```python
from build123d import *

# Parameters (mm, degrees)
SKETCH1_W           = 50
SKETCH1_H           = 50
BOSS_EXTRUDE1_DEPTH = 50
SKETCH2_R           = 20
CUT_EXTRUDE1_DEPTH  = 5
SKETCH3_R           = 20
CUT_EXTRUDE5_DEPTH  = 2
FILLET10_R          = 30
FILLET11_R          = 10
FILLET12_R          = 10
FILLET15_R          = 5
FILLET16_R          = 5


with BuildPart() as part:
    # Sketch1 → Boss-Extrude1 (new body)
    with BuildSketch(Plane(origin=(0, 0, 0), x_dir=(1, 0, 0), z_dir=(0, 1, 0))):
        Rectangle(SKETCH1_W, SKETCH1_H)
    extrude(amount=BOSS_EXTRUDE1_DEPTH)

    # Sketch2 → Cut-Extrude1 (cut)
    with BuildSketch(Plane(origin=(0, 0, -25), x_dir=(-1, 0, 0), z_dir=(0, 0, -1))):
        with Locations((0, 25)):
            Circle(SKETCH2_R)
    extrude(amount=-CUT_EXTRUDE1_DEPTH, mode=Mode.SUBTRACT)

    # Sketch3 → Cut-Extrude5 (cut)
    with BuildSketch(Plane.XZ):
        with Locations(Location((0, 0, 0), (0, 0, 270))):
            Circle(SKETCH3_R)
    extrude(amount=-CUT_EXTRUDE5_DEPTH, mode=Mode.SUBTRACT)

    # Fillet10
    fillet10_edges = [part.edges().sort_by_distance(p)[0] for p in [
        (0, 50, 25),
    ]]
    fillet(fillet10_edges, radius=FILLET10_R)

    # Fillet11
    fillet11_edges = [part.edges().sort_by_distance(p)[0] for p in [
        (25, 50, -15),
        (25, 10, 25),
        (25, 41.213203436, 16.213203436),
    ]]
    fillet(fillet11_edges, radius=FILLET11_R)

    # Fillet12
    fillet12_edges = [part.edges().sort_by_distance(p)[0] for p in [
        (-25, 50, -15),
        (-25, 10, 25),
        (-25, 41.213203436, 16.213203436),
    ]]
    fillet(fillet12_edges, radius=FILLET12_R)

    # Fillet15
    fillet15_edges = [part.edges().sort_by_distance(p)[0] for p in [
        (25, 0, -5),
        (22.071067812, 0, 22.071067812),
        (0, 0, 25),
        (-22.071067812, 0, 22.071067812),
        (-25, 0, -5),
    ]]
    fillet(fillet15_edges, radius=FILLET15_R - 0.0001)  # a hair under: the kernel refuses the full size

    # Fillet16
    fillet16_edges = [part.edges().sort_by_distance(p)[0] for p in [
        (25, 22.49995, -25),
        (0, 50, -25),
        (22.071067812, 47.071067812, -25),
        (-25, 22.49995, -25),
        (-22.071067812, 47.071067812, -25),
        (0, 0, -25),
        (-23.535563195, 1.464436805, -25),
        (23.535563195, 1.464436805, -25),
    ]]
    fillet(fillet16_edges, radius=FILLET16_R - 0.0001)  # a hair under: the kernel refuses the full size


solid = part.part
```
Model file for the job. Use its own axes, mm. A direction names the side the tool comes from. Coordinates: 2 decimals unless noted, no trailing zeros. Order: outer loops, then holes, each group sorted by start corner. A loop starts at its lowest first (then second) coordinate and runs counter-clockwise, first axis right, second up. Notation, with made-up numbers: (8.5, -21) -> (46.5, -21) arc R9 cw to (46.5, -4) -> close; hole circle Ø1 at (26.25, 11). An arc over 180 degrees is marked (long way). Answer as a JSON object with one key per item and string values. Group by question number.
1) Pull direction X, two halves, no side cores. Call faces 1 (the face through (-6, 5.6, -25)), 2 (the face through (-19.524, 0.986, 4.336)), 3 (the face through (-23, 1, -2)): +X half, -X half, draft (parallel to the pull), parting line (faces both ways), or undercut.
2) Which spindle directions (+Z, -Z, +X, -X, +Y, -Y) get a long thin tool onto all of the face, cutting with end or side? Do faces 4 (the face through (0, 2, 0)), 5 (the face through (4.336, 5.476, -22.535)), 6 (the face through (-24, 22, -23)). Say none if no direction does.
3) Cut at A-A, the plane y = 9. Write the cut outline in (x, z), then the cut area to 3 significant figures.
4) Cut at C-C, the plane z = -11. Write the cut outline in (x, y), then the cut area to 3 significant figures.
5) Flat gauge pins, fed straight in: pin 1 (20 mm diameter, centred on x = -3.5, z = -5, fed in from -Y); pin 2 (2 mm diameter, centred on y = 38, z = 15.5, fed in from -X). Where does each tip first touch, or does it go through?
6) Cut at D-D, the plane x = -13. Write the cut outline in (y, z), then the cut area to 3 significant figures.
7) Drill centre lines: L1, parallel to Y at x = 0, z = -22; L2, parallel to Z at x = 12, y = 15; L3, parallel to Y at x = 4, z = -4. Where is each one in solid material? Low to high.
Check values:
{
 "1": {"face 1": "draft", "face 2": "undercut", "face 3": "-X half"},
 "2": {"face 4": "-Y", "face 5": "-Z", "face 6": "-Z, -X, +Y, -Y"},
 "3": {"outline": "(-25, -20) arc R5 ccw to (-20, -25) -> (-12, -25) -> (-12, -20) -> (12, -20) -> (12, -25) -> (20, -25) arc R5 ccw to (25, -20) -> (25, 15) arc R10 ccw to (15, 25) -> (-15, 25) arc R10 ccw to (-25, 15) -> close", "area": "2,330 mm²"},
 "4": {"outline": "(-25, 5) arc R5 ccw to (-20, 0) -> (-16.7, 0) -> (-16.7, 2) -> (16.7, 2) -> (16.7, 0) -> (20, 0) arc R5 ccw to (25, 5) -> (25, 40) arc R10 ccw to (15, 50) -> (-15, 50) arc R10 ccw to (-25, 40) -> close", "area": "2,380 mm²"},
 "5": {"pin 1": "stops at y = 2", "pin 2": "stops at x = -22.78"},
 "6": {"outline": "(0, -20) arc R5 ccw to (5, -25) -> (9.8, -25) -> (9.8, -20) -> (40.2, -20) -> (40.2, -25) -> (45, -25) arc R5 ccw to (50, -20) -> (50, -5) arc R30 ccw to (20, 25) -> (5, 25) arc R5 ccw to (0, 20) -> (0, 15.2) -> (2, 15.2) -> (2, -15.2) -> (0, -15.2) -> close", "area": "2,080 mm²"},
 "7": {"L1": "y = 0.42 to 5, 45 to 49.58", "L2": "z = -20 to 25", "L3": "y = 2 to 49.98"}
}
